Autodesk Inventor part; units mm, degrees
ref_plane "YZ Plane" through (0, 0, 0) normal (1, 0, 0) x (0, 1, 0)
ref_plane "XZ Plane" through (0, 0, 0) normal (0, 1, 0) x (-1, 0, 0)
ref_plane "XY Plane" through (0, 0, 0) normal (0, 0, 1) x (1, 0, 0)
sketch "Sketch1" plane through (0, 0, 0) normal (0, 0, 1) x (1, 0, 0)
  arc A0 (0, 12) -> (8, 14.5109) centre (0, 26) ccw
  line L0 (0, 0) -> (0, 12) construction
  line L1 (8, 14.5109) -> (8, 0)
  arc A1 (-8, 14.5109) -> (0, 12) centre (0, 26) ccw
  line L2 (-8, 14.5109) -> (-8, 0)
  line L3 (-8, 0) -> (0, 0)
  line L4 (0, 0) -> (8, 0)
  dimension "d0" = 14
  dimension "d9" = 8
  dimension "d13" = 26
extrude "Extrusion1" add sketch "Sketch1" along normal blind 10
sketch "Sketch2" plane through (-8, 0, 0) normal (0, -1, 0) x (1, 0, 0)
  circle A0 centre (-10, 16) radius 2
  circle A1 centre (26, 16) radius 2
  line L0 (-10, 16) -> (26, 16) construction
  line L1 (16, 0) -> (0, 0) construction
  line L2 (0, 10) -> (16, 10) construction
  line L3 (-15, 22) -> (31, 22)
  line L4 (31, 22) -> (31, 10)
  line L5 (31, 10) -> (-15, 10)
  line L6 (-15, 10) -> (-15, 22)
  point P0 (8, 0)
  point P1 (8, 16)
  point P2 (8, 0)
  point P3 (31, 16)
  point P4 (8, 22)
  dimension "d14" = 4
  dimension "d15" = 4
  dimension "d16" = 36
  dimension "d17" = 6
  dimension "d18" = 46
extrude "Extrusion2" add sketch "Sketch2" against normal blind 3
fillet "Fillet1" radius 6 1 edges at (0, 3, 10)
properties part number "DefaultMotorMountBack" material "ABS Plastic"
Build history of the part. All positions in model axes, mm. A direction names the side the tool comes from. Give positions to 0.01 mm unless a question says otherwise; leave off trailing zeros. Loops run counter-clockwise (first coordinate to the right, second up) from the corner with the lowest first, then second, coordinate; pieces in that order, holes last.
1) 3-axis set-ups, long thin cutter, end or side, ignore diameter. For faces 4 (the face through (0, 11, 10)), 5 (the face through (16, 1, 10)), 6 (the face through (-4.135, 12.625, 4.93)): which of +Z, -Z, +X, -X, +Y, -Y reach the whole face in a straight line?
Values follow:
face 4: +Z, +X, -X, +Y
face 5: -Z, +X, +Y, -Y
face 6: +Z, -Z, +Y
2) Band-saw the part on A-A on y = 1. List the corners of the cut face in (x, z), then the cut area to 3 significant figures.
Values follow:
outline: (-23, 10) - (-8, 10) - (-8, 0) - (8, 0) - (8, 10) - (23, 10) - (23, 22) - (-23, 22) - close; hole circle Ø4 at (-18, 16); hole circle Ø4 at (18, 16)
area: 687 mm2
3) Probe line 1 along Z through (x, y) = (18, 1.25); line 2 along Y through (x, z) = (2, 19.75); line 3 along X through (y, z) = (10.75, 9.5). List the from-to ranges inside material, lowest first.
Values follow:
line 1: z = 10 to 14, 18 to 22
line 2: y = 0 to 3
line 3: x = -8 to 8
4) Drop flat-ended pins along their axis: P1, Ø1.5, axis at x = -12.5, y = 1.5, coming from the -Z side; P2, Ø4, axis at y = 7, z = 6.5, coming from the -X side; P3, Ø6, axis at x = 7, z = 15, coming from the +Y side; P4, Ø1, axis at x = 1.5, y = 11.5, coming from the -Z side. Give the stop position or say it passes through.
Values follow:
P1: stops at z = 10
P2: stops at x = -8
P3: stops at y = 4.53
P4: stops at z = 0
5) Two-plate mould, pull along X, no slides. Class faces 1 (the face through (0, 1, 22)), 2 (the face through (18, 1, 18)), 3 (the face through (23, 1, 16)): released by +X, released by -X, zero draft, split by the parting line, or undercut.
Values follow:
face 1: zero draft
face 2: undercut
face 3: released by +X
6) Band-saw the part on B-B on x = -18. List the corners of the cut face in (y, z).
Values follow:
outline: (0, 10) - (3, 10) - (3, 14) - (0, 14) - close; (0, 18) - (3, 18) - (3, 22) - (0, 22) - close
7) Band-saw the part on D-D on z = 15.5. State how many separate pieces and enclosed holes the cut face has, then the cut area to 3 significant figures.
Values follow:
separate pieces: 3
enclosed holes: 0
area: 115 mm2
8) Band-saw the part on C-C on z = 5.75. List the corners of the cut face in (x, y), then the cut area to 3 significant figures.
Values follow:
outline: (-8, 0) - (8, 0) - (8, 14.51) arc R14 cw to (0, 12) arc R14 cw to (-8, 14.51) - close
area: 205 mm2
